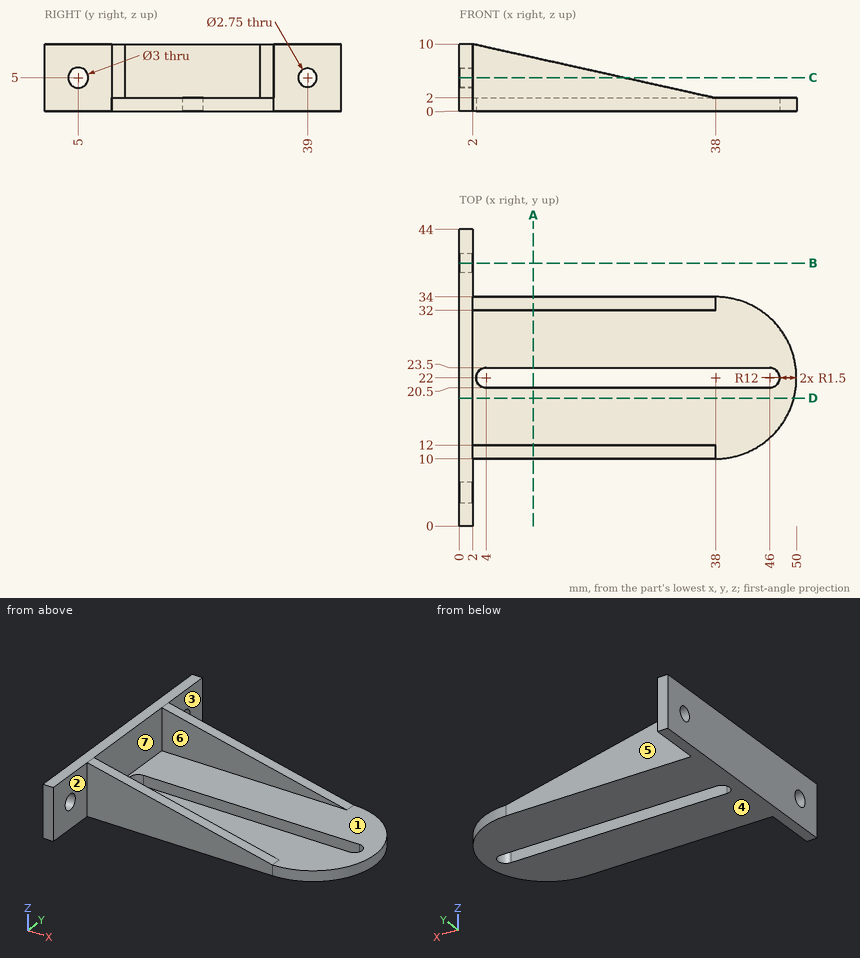
Study the drawing (mm; zero at the part's minimum x, y, z) and answer. A direction names the side the tool comes from. Coordinates: 2 decimals unless noted, no trailing zeros. Write each loop counter-clockwise with the first axis right and the second up, starting at its lowest first coordinate (ties: lowest second). Pieces come first, ordered by that corner, then holes. Notation, with made-up numbers: (30, 75.25) -> (82, 75.25) arc R29 cw to (82, 109.25) -> close; hole circle Ø2 at (67.25, 4.5). An arc over 180 degrees is marked (long way). Write item = value, one per line.
(1) Section A-A on x = 11 is taken. Write down the section's boundary in (y, z), plus the area to 3 significant figures.
From the geometry:
outline = (10, 0) -> (20.5, 0) -> (20.5, 2) -> (12, 2) -> (12, 8) -> (10, 8) -> close; (23.5, 0) -> (34, 0) -> (34, 8) -> (32, 8) -> (32, 2) -> (23.5, 2) -> close
area = 66.0 mm2
(2) Given pin 1 Ø1 at (y, z) = (39, 4.5) entering from +X; pin 2 Ø1 at (x, z) = (17.5, 7) entering from -Y; pin 3 Ø1 at (x, z) = (24, 0.5) entering from +Y, each flat-ended and moving along its own axis, determine where each tip first touches the part or whether it passes through.
From the geometry:
pin_1 = through
pin_2 = 10
pin_3 = 34
(3) Section C-C on z = 5 is taken. Write down the section's boundary in (x, y) (3 decimals).
From the geometry:
outline = (0, 0) -> (2, 0) -> (2, 3.5) -> (0, 3.5) -> close; (0, 6.5) -> (2, 6.5) -> (2, 10) -> (24.5, 10) -> (24.5, 12) -> (2, 12) -> (2, 32) -> (24.5, 32) -> (24.5, 34) -> (2, 34) -> (2, 37.625) -> (0, 37.625) -> close; (0, 40.375) -> (2, 40.375) -> (2, 44) -> (0, 44) -> close
(4) Section D-D on y = 19 is taken. Write down the section's boundary in (x, z), plus the area to 3 significant figures.
From the geometry:
outline = (0, 0) -> (49.62, 0) -> (49.62, 2) -> (2, 2) -> (2, 10) -> (0, 10) -> close
area = 115 mm2
(5) Which of the six approach directions +Z, -Z, +X, -X, +Y, -Y give full straight-line access (tool end or side, diameter ignored) to the marked faces 1, 2 and 3?
From the geometry:
face_1 = +Z, +X
face_2 = +Z, -Z, +X, -Y
face_3 = +Z, -Z, +X, +Y
(6) Straight lines are drawn through the part: L1, parallel to Y at x = 14, z = 5.5; L2, parallel to X at y = 37.5, z = 6. For each, find the intervals that lie inside material, in ascending order. Write a range as from..to.
From the geometry:
L1 = 10..12, 32..34
L2 = 0..2
(7) For a pull along Y with two mould halves and no side action, classify the marked faces 4, 5, 6 and 7 as +Y half, -Y half, draft (parallel to the pull), parting line (faces both ways), or undercut.
From the geometry:
face_4 = draft
face_5 = +Y half
face_6 = undercut
face_7 = undercut
(8) Section B-B on y = 39 is taken. Write down the section's boundary in (x, z) (3 decimals).
From the geometry:
outline = (0, 0) -> (2, 0) -> (2, 3.625) -> (0, 3.625) -> close; (0, 6.375) -> (2, 6.375) -> (2, 10) -> (0, 10) -> close
